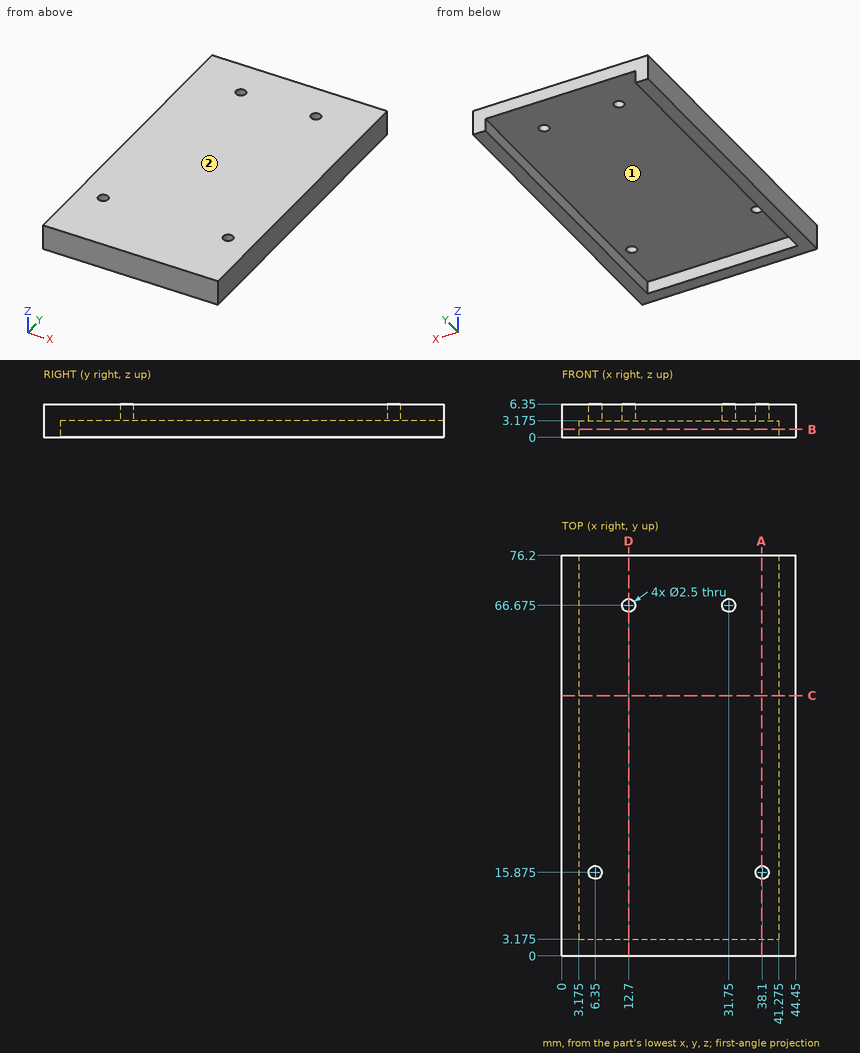
Could you check a few things on this drawing? It's one solid part, dimensions in mm from its lowest x, y, z. A direction names the side the tool comes from. Give positions to 0.01 mm unless a question says otherwise; leave off trailing zeros. Order: outer loops, then holes, each group sorted by start corner. A loop starts at its lowest first (then second) coordinate and runs counter-clockwise, first axis right, second up. Notation, with made-up numbers: (72, 27) - (116, 27) arc R21 ccw to (116, 42) - close; hole circle Ø1 at (72, 33). An arc over 180 degrees is marked (long way). One line per item, written item: value. Start each with the question number.
1. Imagine slicing it at A-A on x = 38. List the corners of the cut face in (y, z) for me (3 decimals), plus the area to 3 significant figures.
2. Imagine slicing it at C-C on y = 49.5. List the corners of the cut face in (x, z) for me (3 decimals).
3. Imagine slicing it at D-D on x = 12.7. List the corners of the cut face in (y, z) for me (3 decimals).
4. Imagine slicing it at B-B on z = 1.5. List the corners of the cut face in (x, y) for me (3 decimals).
5. For P1, Ø2.5, axis at x = 31, z = 1, coming from the +Y side (3 decimals); P2, Ø3, axis at y = 66, z = 4, coming from the -X side; P3, Ø10, axis at x = 11, y = 68, coming from the -Z side (3 decimals), each with a flat end and sliding along its axis, tell me the tip position at first contact or that it passes through.
6. If I drill on probe 1 along X at (y, z) = (32, 2.25) (3 decimals); probe 2 along Y at (x, z) = (6.35, 5.15) (3 decimals); probe 3 along Y at (x, z) = (31.75, 5.15) (3 decimals), over which ranges is the centre line in solid material (lowest first)?
7. For the marked faces 1 and 2, which set-ups out of +Z, -Z, +X, -X, +Y, -Y let a thin tool reach every point of the face, with its end or its side?
Values:
1. outline: (0, 0) - (3.175, 0) - (3.175, 3.175) - (14.629, 3.175) - (14.629, 6.35) - (0, 6.35) - close; (17.121, 3.175) - (76.2, 3.175) - (76.2, 6.35) - (17.121, 6.35) - close
1. area: 244 mm²
2. outline: (0, 0) - (3.175, 0) - (3.175, 3.175) - (41.275, 3.175) - (41.275, 0) - (44.45, 0) - (44.45, 6.35) - (0, 6.35) - close
3. outline: (0, 0) - (3.175, 0) - (3.175, 3.175) - (65.425, 3.175) - (65.425, 6.35) - (0, 6.35) - close; (67.925, 3.175) - (76.2, 3.175) - (76.2, 6.35) - (67.925, 6.35) - close
4. outline: (0, 0) - (44.45, 0) - (44.45, 76.2) - (41.275, 76.2) - (41.275, 3.175) - (3.175, 3.175) - (3.175, 76.2) - (0, 76.2) - close
5. P1: y = 3.175
5. P2: x = 0
5. P3: z = 3.175
6. probe 1: 0 to 3.175, 41.275 to 44.45
6. probe 2: 0 to 14.625, 17.125 to 76.2
6. probe 3: 0 to 65.425, 67.925 to 76.2
7. face 1: -Z, +Y
7. face 2: +Z, +X, -X, +Y, -Y
